Source: CAD feature listing. Evaluate the final solid. Frame: model axes, mm. A direction names the side the tool comes from. Round coordinates to 2 decimals unless told otherwise and drop trailing zeros. Write each loop counter-clockwise with the first axis right and the second up, starting at its lowest first coordinate (ties: lowest second). Pieces come first, ordered by that corner, then holes.
from build123d import *

# Parameters (mm, degrees)
SKETCH_1_R          = 22
EXTRUDE_1_DEPTH     = 2
SKETCH_2_R          = 2
SKETCH_2_R_2        = 0.6
EXTRUDE_2_DEPTH     = 4
SKETCH_3_R          = 25
EXTRUDE_3_DEPTH     = 2
CUT_EXTRUDE_2_DEPTH = 1
SKETCH_6_R          = 5.45
SKETCH_6_R_2        = 3.85
CUT_EXTRUDE_3_DEPTH = 1.3
SKETCH_8_R          = 0.6
CUT_EXTRUDE_4_DEPTH = 18.5
SKETCH_9_R          = 16.695755265
CUT_EXTRUDE_5_DEPTH = 2
SKETCH_10_R         = 1.6
CUT_EXTRUDE_6_DEPTH = 1
SKETCH_11_R         = 1.6
CUT_EXTRUDE_7_DEPTH = 3
SKETCH_13_R         = 2
SKETCH_13_R_2       = 0.6
EXTRUDE_4_DEPTH     = 2
SKETCH_14_R         = 0.8
CUT_EXTRUDE_8_DEPTH = 10


with BuildPart() as part:
    # 草图1 → 凸台-拉伸1 (new body)
    with BuildSketch(Plane.XY):
        Circle(SKETCH_1_R)
    extrude(amount=EXTRUDE_1_DEPTH)

    # 草图2 → 凸台-拉伸2 (add)
    with BuildSketch(Plane.XY.offset(2)):
        with Locations((-10, 0)):
            Circle(SKETCH_2_R)
        with Locations((-10, 0)):
            Circle(SKETCH_2_R_2, mode=Mode.SUBTRACT)
        with Locations((5, 8.660254038)):
            Circle(SKETCH_2_R)
        with Locations((5, 8.660254038)):
            Circle(SKETCH_2_R_2, mode=Mode.SUBTRACT)
        with Locations((5, -8.660254038)):
            Circle(SKETCH_2_R)
        with Locations((5, -8.660254038)):
            Circle(SKETCH_2_R_2, mode=Mode.SUBTRACT)
    extrude(amount=EXTRUDE_2_DEPTH)

    # 草图3 → 凸台-拉伸3 (add)
    with BuildSketch(Plane(origin=(0, 0, 0), x_dir=(-1, 0, 0), z_dir=(0, 0, -1))):
        Circle(SKETCH_3_R)
    extrude(amount=EXTRUDE_3_DEPTH)

    # 草图5 → 切除-拉伸2 (cut)
    with BuildSketch(Plane(origin=(0, 0, -2), x_dir=(-1, 0, 0), z_dir=(0, 0, -1))):
        Polygon((21, -3.95), (21, -4), (29.149006969, -4), (29.149006969, 4), (21, 4), align=None)
    extrude(amount=-CUT_EXTRUDE_2_DEPTH, mode=Mode.SUBTRACT)

    # 草图6 → 切除-拉伸3 (cut)
    with BuildSketch(Plane(origin=(0, 0, -2), x_dir=(-1, 0, 0), z_dir=(0, 0, -1))):
        with Locations((-18, 0)):
            Circle(SKETCH_6_R)
        with Locations((-18, 0)):
            Circle(SKETCH_6_R_2, mode=Mode.SUBTRACT)
        with Locations((9, 15.588457268)):
            Circle(SKETCH_6_R)
        with Locations((9, 15.588457268)):
            Circle(SKETCH_6_R_2, mode=Mode.SUBTRACT)
        with Locations((9, -15.588457268)):
            Circle(SKETCH_6_R)
        with Locations((9, -15.588457268)):
            Circle(SKETCH_6_R_2, mode=Mode.SUBTRACT)
    extrude(amount=-CUT_EXTRUDE_3_DEPTH, mode=Mode.SUBTRACT)

    # 草图8 → 切除-拉伸4 (cut)
    with BuildSketch(Plane.XY.offset(6)):
        with Locations((5, -8.660254038)):
            Circle(SKETCH_8_R)
        with Locations((-10, 0)):
            Circle(SKETCH_8_R)
        with Locations((5, 8.660254038)):
            Circle(SKETCH_8_R)
    extrude(amount=-CUT_EXTRUDE_4_DEPTH, mode=Mode.SUBTRACT)

    # 草图9 → 切除-拉伸5 (cut)
    with BuildSketch(Plane.XY.offset(6)):
        Circle(SKETCH_9_R)
    extrude(amount=-CUT_EXTRUDE_5_DEPTH, mode=Mode.SUBTRACT)

    # 草图10 → 切除-拉伸6 (cut)
    with BuildSketch(Plane(origin=(0, 0, -2), x_dir=(-1, 0, 0), z_dir=(0, 0, -1))):
        with Locations((-5, -8.660254038)):
            Circle(SKETCH_10_R)
        with Locations((-5, 8.660254038)):
            Circle(SKETCH_10_R)
    extrude(amount=-CUT_EXTRUDE_6_DEPTH, mode=Mode.SUBTRACT)

    # 草图11 → 切除-拉伸7 (cut)
    with BuildSketch(Plane(origin=(0, 0, -2), x_dir=(-1, 0, 0), z_dir=(0, 0, -1))):
        with Locations((10, 0)):
            Circle(SKETCH_11_R)
    extrude(amount=-CUT_EXTRUDE_7_DEPTH, mode=Mode.SUBTRACT)

    # 草图13 → 凸台-拉伸4 (add)
    with BuildSketch(Plane.XY.offset(4)):
        with Locations((-10, 0)):
            Circle(SKETCH_13_R)
        with Locations((-10, 0)):
            Circle(SKETCH_13_R_2, mode=Mode.SUBTRACT)
        with Locations((5, 8.660254038)):
            Circle(SKETCH_13_R)
        with Locations((5, 8.660254038)):
            Circle(SKETCH_13_R_2, mode=Mode.SUBTRACT)
        with Locations((5, -8.660254038)):
            Circle(SKETCH_13_R)
        with Locations((5, -8.660254038)):
            Circle(SKETCH_13_R_2, mode=Mode.SUBTRACT)
    extrude(amount=EXTRUDE_4_DEPTH)

    # 草图14 → 切除-拉伸8 (cut)
    with BuildSketch(Plane(origin=(0, 0, -2), x_dir=(-1, 0, 0), z_dir=(0, 0, -1))):
        with Locations((-2.664556788, 3.004852263)):
            Circle(SKETCH_14_R)
        with Locations((-0.464852263, 1.734852263)):
            Circle(SKETCH_14_R)
        with Locations((1.734852263, 0.464852263)):
            Circle(SKETCH_14_R)
        with Locations((3.934556788, -0.805147737)):
            Circle(SKETCH_14_R)
        with Locations((-1.734852263, -0.464852263)):
            Circle(SKETCH_14_R)
        with Locations((0.464852263, -1.734852263)):
            Circle(SKETCH_14_R)
        with Locations((2.664556788, -3.004852263)):
            Circle(SKETCH_14_R)
        with Locations((-3.934556788, 0.805147737)):
            Circle(SKETCH_14_R)
    extrude(amount=-CUT_EXTRUDE_8_DEPTH, mode=Mode.SUBTRACT)


solid = part.part
1) Section query A-A on z = 4.75. Return the cut outline in (x, y), then the cut area to 3 significant figures.
Taken from the geometry:
outline: circle Ø4 at (-10, 0); circle Ø4 at (5, -8.66); circle Ø4 at (5, 8.66); hole circle Ø1.2 at (-10, 0); hole circle Ø1.2 at (5, -8.66); hole circle Ø1.2 at (5, 8.66)
area: 34.3 mm2
2) Contact query for flat-ended pins moving along their axis: P1, Ø1.5, axis at x = 9.5, y = 15.5, coming from the +Z side; P2, Ø1.5, axis at y = -3, z = 0.5, coming from the +X side; P3, Ø1, axis at x = -19.5, y = 14.5, coming from the +Z side; P4, Ø1, axis at x = -2.66, y = -3, coming from the +Z side. Output: stop coordinate, or through.
Taken from the geometry:
P1: stops at z = 2
P2: stops at x = 24.88
P3: stops at z = 0
P4: passes through
3) Material intervals for line 1 (Y direction, x = 5, z = 4.65); line 2 (Y direction, x = -10, z = 2.35); line 3 (X direction, y = -18.5, z = -0.75), sorted ascending.
Taken from the geometry:
line 1: y = -10.66 to -9.26, -8.06 to -6.66, 6.66 to 8.06, 9.26 to 10.66
line 2: y = -2 to -0.6, 0.6 to 2
line 3: x = -16.82 to -13.61, -11.52 to -6.48, -4.39 to 16.82
4) Reachability of faces 1 (the face through (-5, 14, -0.7)), 2 (the face through (-4.769, -21.477, 0.986)), 3 (the face through (-23.846, 7.509, -0.986)), 4 (the face through (-23, 0, -1)) from +Z, -Z, +X, -X, +Y, -Y: full face, straight path, thin tool, end or side. Return the list, or none.
Taken from the geometry:
face 1: -Z
face 2: +Z
face 3: +Z, -Z
face 4: -Z, -X
5) Section query D-D on x = 10. Return the cut outline in (y, z), then the cut area to 3 significant figures.
Taken from the geometry:
outline: (-22.91, -2) - (22.91, -2) - (22.91, 0) - (19.6, 0) - (19.6, 2) - (-19.6, 2) - (-19.6, 0) - (-22.91, 0) - close
area: 170 mm2
6) Section query B-B on x = 18. Return the cut outline in (y, z), then the cut area to 3 significant figures.
Taken from the geometry:
outline: (-17.35, -2) - (-5.45, -2) - (-5.45, -0.7) - (-3.85, -0.7) - (-3.85, -2) - (3.85, -2) - (3.85, -0.7) - (5.45, -0.7) - (5.45, -2) - (17.35, -2) - (17.35, 0) - (12.65, 0) - (12.65, 2) - (-12.65, 2) - (-12.65, 0) - (-17.35, 0) - close
area: 116 mm2
7) Pull-direction query (X, two-part tool) for faces 5 (the face through (0.5, 0.4, -2)), 6 (the face through (0.972, -0.225, -0.028)), 7 (the face through (-10, -1, 1)), 8 (the face through (-11.6, -1.2, 4)); classes: released by +X, released by -X, zero draft, split by the parting line, or undercut.
Taken from the geometry:
face 5: zero draft
face 6: undercut
face 7: undercut
face 8: split by the parting line
8) Section query C-C on y = -15. Return the cut outline in (x, z), then the cut area to 3 significant figures.
Taken from the geometry:
outline: (-20, -2) - (-14.42, -2) - (-14.42, -0.7) - (-12.8, -0.7) - (-12.8, -2) - (-5.2, -2) - (-5.2, -0.7) - (-3.58, -0.7) - (-3.58, -2) - (20, -2) - (20, 0) - (16.09, 0) - (16.09, 2) - (-16.09, 2) - (-16.09, 0) - (-20, 0) - close
area: 140 mm2
